Part model, mm, in its own coordinate system. A direction names the side the tool comes from. Give positions to 0.01 mm unless a question says otherwise; leave off trailing zeros. Write each loop counter-clockwise with the first axis right and the second up, starting at its lowest first coordinate (ties: lowest second). Pieces come first, ordered by that corner, then holes.
from build123d import *

# Parameters (mm, degrees)
SKETCH005_W  = 85
SKETCH005_H  = 56
SKETCH005_R  = 1.5
PAD003_DEPTH = 1.4
SKETCH009_W  = 20
SKETCH009_H  = 56
PAD007_DEPTH = 16
SKETCH010_W  = 30
SKETCH010_H  = 15
PAD008_DEPTH = 1
SKETCH011_W  = 9
SKETCH011_H  = 7.5
PAD009_DEPTH = 3.2
PAD010_DEPTH = 50


with BuildPart() as part:
    # Sketch005 → Pad003 (new body)
    with BuildSketch(Plane.XY):
        with Locations((42.5, 28)):
            Rectangle(SKETCH005_W, SKETCH005_H)
        with Locations((23.5, 52.5)):
            Circle(SKETCH005_R, mode=Mode.SUBTRACT)
        with Locations((23.5, 3.5)):
            Circle(SKETCH005_R, mode=Mode.SUBTRACT)
        with Locations((81.5, 52.5)):
            Circle(SKETCH005_R, mode=Mode.SUBTRACT)
        with Locations((81.5, 3.5)):
            Circle(SKETCH005_R, mode=Mode.SUBTRACT)
    extrude(amount=PAD003_DEPTH)

    # Sketch009 → Pad007 (join)
    with BuildSketch(Plane.XY.offset(1.4)):
        with Locations((7, 28)):
            Rectangle(SKETCH009_W, SKETCH009_H)
    extrude(amount=PAD007_DEPTH)

    # Sketch010 → Pad008 (join)
    with BuildSketch(Plane.XY):
        with Locations((73, 28)):
            Rectangle(SKETCH010_W, SKETCH010_H)
    extrude(amount=-PAD008_DEPTH)

    # Sketch011 → Pad009 (join)
    with BuildSketch(Plane.XY.offset(1.4)):
        with Locations((73.8, 53.75)):
            Rectangle(SKETCH011_W, SKETCH011_H)
    extrude(amount=PAD009_DEPTH)

    # Sketch013 → Pad010 (join)
    with BuildSketch(Plane.XY):
        Polygon((41.5, 55), (41.5, 33), (38.5, 33), (38.5, 55), (40, 55), align=None)
    extrude(amount=PAD010_DEPTH)


solid = part.part
1) Saw through at A-A (y = 3.5). Write the cut outline in (x, z), and give its area (3 significant figures).
Check result:
outline: (-3, 1.4) - (0, 1.4) - (0, 0) - (22, 0) - (22, 1.4) - (17, 1.4) - (17, 17.4) - (-3, 17.4) - close; (25, 0) - (80, 0) - (80, 1.4) - (25, 1.4) - close; (83, 0) - (85, 0) - (85, 1.4) - (83, 1.4) - close
area: 431 mm2
2) 3-axis set-ups, long thin cutter, end or side, ignore diameter. For faces 4 (the flat face through (74, 50, 3)), 5 (the flat face through (7, 28, 17.4)), 6 (the flat face through (-2, 28, 1.4)), 7 (the flat face through (78.3, 54, 3)), 8 (the flat face through (69.3, 54, 3)): which of +Z, -Z, +X, -X, +Y, -Y reach the whole face in a straight line?
Check result:
face 4: +Z, +X, -Y
face 5: +Z, -X, +Y, -Y
face 6: -Z, -X, +Y, -Y
face 7: +Z, +X, +Y, -Y
face 8: +Z, +Y, -Y
3) Saw through at B-B (x = 23.5). Write the cut outline in (y, z).
Check result:
outline: (0, 0) - (2, 0) - (2, 1.4) - (0, 1.4) - close; (5, 0) - (51, 0) - (51, 1.4) - (5, 1.4) - close; (54, 0) - (56, 0) - (56, 1.4) - (54, 1.4) - close
4) Saw through at C-C (x = 81.5). Write the cut outline in (y, z), and give its area (3 significant figures).
Check result:
outline: (0, 0) - (2, 0) - (2, 1.4) - (0, 1.4) - close; (5, 0) - (20.5, 0) - (20.5, -1) - (35.5, -1) - (35.5, 0) - (51, 0) - (51, 1.4) - (5, 1.4) - close; (54, 0) - (56, 0) - (56, 1.4) - (54, 1.4) - close
area: 85.0 mm2
5) Saw through at D-D (z = 43). Write the cut outline in (x, y), and give its area (3 significant figures).
Check result:
outline: (38.5, 33) - (41.5, 33) - (41.5, 55) - (38.5, 55) - close
area: 66.0 mm2
6) Mould opens along X. For faces 1 (the flat face through (-3, 28, 9)), 2 (the flat face through (51, 28, 1.4)), 3 (the flat face through (74, 54, 4.6)) say: +X half, -X half, draft (parallel to the pull), parting line (faces both ways), or undercut.
Check result:
face 1: -X half
face 2: undercut
face 3: draft
7) Drill centre lines: L1, parallel to Y at x = 23.5, z = 0.3; L2, parallel to Y at x = 81, z = 1; L3, parallel to X at y = 17.5, z = 9.5. Where is each one in solid material? Low to high.
Check result:
L1: y = 0 to 2, 5 to 51, 54 to 56
L2: y = 0 to 2.09, 4.91 to 51.09, 53.91 to 56
L3: x = -3 to 17
8) Flat gauge pins, fed straight in: P1, Ø6, axis at x = 36.5, z = 34, coming from the -Y side; P2, Ø2.5, axis at x = 23.5, y = 52.5, coming from the +Z side; P3, Ø2.5, axis at y = 54.5, z = 3.5, coming from the +X side; P4, Ø24, axis at y = 38.5, z = 24, coming from the -X side. Where does each tip first touch, or does it go through?
Check result:
P1: stops at y = 33
P2: passes through
P3: stops at x = 78.3
P4: stops at x = -3
